For this review, take the finished solid that the model builds, in its own axes (mm). Coordinates: 2 decimals unless noted, no trailing zeros. Loops run counter-clockwise (first coordinate to the right, second up) from the corner with the lowest first, then second, coordinate; pieces in that order, holes last. Notation, with made-up numbers: M 21,86 L 68,86 A12 cw 68,107 Z; hole C -9.75,26.25 d5. An arc over 180 degrees is marked long. Put each result on its own line as item: value.
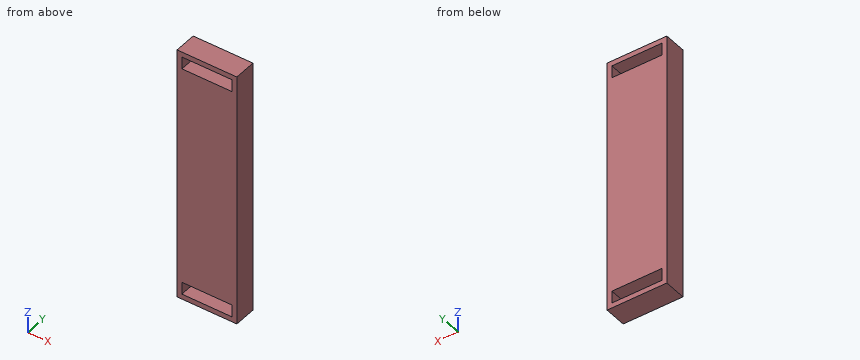
Autodesk Inventor part; units mm, degrees
ref_plane "YZ Plane" through (0, 0, 0) normal (1, 0, 0) x (0, 1, 0)
ref_plane "XZ Plane" through (0, 0, 0) normal (0, 1, 0) x (-1, 0, 0)
ref_plane "XY Plane" through (0, 0, 0) normal (0, 0, 1) x (1, 0, 0)
sketch "Sketch1" plane through (0, 0, 0) normal (0, 0, 1) x (1, 0, 0)
  line L0 (-17.5, 6.5) -> (17.5, 6.5)
  line L1 (17.5, 6.5) -> (17.5, -6.5)
  line L2 (17.5, -6.5) -> (-17.5, -6.5)
  line L3 (-17.5, -6.5) -> (-17.5, 6.5)
  line L4 (-17.5, 6.5) -> (17.5, -6.5) construction
  line L5 (17.5, 6.5) -> (-17.5, -6.5) construction
  line L6 (-17.5, 6.5) -> (17.5, 6.5) construction
  point P0 (0, 0)
  dimension "d0" = 35
  dimension "d1" = 0
  dimension "d2" = 13
extrude "Extrusion1" add sketch "Sketch1" along normal blind 150
sketch "Sketch2" plane through (-17.5, 6.5, 0) normal (0, 1, 0) x (1, 0, 0)
  line L0 (2.8, -10.2) -> (32.2, -10.2)
  line L1 (32.2, -10.2) -> (32.2, -3)
  line L2 (32.2, -3) -> (2.8, -3)
  line L3 (2.8, -3) -> (2.8, -10.2)
  line L4 (2.8, -10.2) -> (32.2, -3) construction
  line L5 (32.2, -10.2) -> (2.8, -3) construction
  line L6 (2.8, -10.2) -> (32.2, -10.2) construction
  line L7 (2.8, -6.6) -> (0, -6.6)
  line L8 (0, 0) -> (0, -150)
  line L9 (35, 0) -> (35, -150)
  line L10 (35, -6.6) -> (32.2, -6.6)
  line L11 (35, 0) -> (0, 0)
  line L12 (2.8, -147) -> (32.2, -147)
  line L13 (32.2, -147) -> (32.2, -139.8)
  line L14 (32.2, -139.8) -> (2.8, -139.8)
  line L15 (2.8, -139.8) -> (2.8, -147)
  line L16 (2.8, -147) -> (32.2, -139.8) construction
  line L17 (32.2, -147) -> (2.8, -139.8) construction
  line L18 (2.8, -147) -> (32.2, -147) construction
  line L19 (2.8, -143.4) -> (0, -143.4)
  line L20 (35, -143.4) -> (32.2, -143.4)
  line L21 (35, -150) -> (0, -150)
  point P0 (17.5, 0)
  point P1 (17.5, -6.6)
  point P2 (17.5, -143.4)
  dimension "d6" = 29.4
  dimension "d8" = 7.2
  dimension "d9" = 3
  dimension "d12" = 29.4
  dimension "d13" = 0
  dimension "d14" = 7.2
  dimension "d15" = 3
extrude "Extrusion2" cut sketch "Sketch2" against normal through all contours L3 L2 L1 L0 | L15 L14 L13 L12
properties part number "Leg"
(1) Wall thickness on line 1 along Z through (x, y) = (9, 2); line 2 along X through (y, z) = (0.5, 7.5): over which ranges is each line inside the solid? List them lowest first. Write a range as [from, to].
Determined:
line 1: z = [0, 3], [10.2, 139.8], [147, 150]
line 2: x = [-17.5, -14.7], [14.7, 17.5]
(2) Add section A-A (x = -11). Write out the cut boundary in (y, z).
Determined:
outline: M -6.5,0 L 6.5,0 L 6.5,3 L -6.5,3 Z; M -6.5,10.2 L 6.5,10.2 L 6.5,139.8 L -6.5,139.8 Z; M -6.5,147 L 6.5,147 L 6.5,150 L -6.5,150 Z
(3) Add section B-B (y = 0.5). Write out the cut boundary in (x, z), plus the area to 3 significant figures.
Determined:
outline: M -17.5,0 L 17.5,0 L 17.5,150 L -17.5,150 Z; hole M -14.7,3 L 14.7,3 L 14.7,10.2 L -14.7,10.2 Z; hole M -14.7,139.8 L 14.7,139.8 L 14.7,147 L -14.7,147 Z
area: 4,830 mm^2
